Part model, mm, in its own coordinate system. A direction names the side the tool comes from. Coordinates: 2 decimals unless noted, no trailing zeros. Loops run counter-clockwise (first coordinate to the right, second up) from the corner with the lowest first, then second, coordinate; pieces in that order, holes last. Notation, with made-up numbers: M -39,-20 L -21,-20 A10 ccw -21,-12 Z; hole C -32,17.25 d8. An arc over 180 degrees is marked long. Answer as CSV lines item,"result". Start each with the question number.
from build123d import *

# Parameters (mm, degrees)
SKETCH061_W     = 19.99996
SKETCH061_H     = 48.49876
SKETCH061_R     = 1.7
PAD018_DEPTH    = 2.54
SKETCH038_W     = 20
SKETCH038_H     = 22.225
PAD004_DEPTH    = 1.5875
POCKET005_DEPTH = 12.7
POCKET006_DEPTH = 9.525
CHAMFER_SIZE    = 1.4986
SKETCH062_R     = 0.9
PAD019_DEPTH    = 2.975
CHAMFER002_SIZE = 1.016
CHAMFER005_SIZE = 1.58496


with BuildPart() as part:
    # Sketch061 → Pad018 (new body)
    with BuildSketch(Plane(origin=(0, 10, -45.999574), x_dir=(-1, 0, 0), z_dir=(0, 1, 0))):
        with Locations((0, 13.85062)):
            Rectangle(SKETCH061_W, SKETCH061_H)
        with Locations((-7.5, 5.00124)):
            Circle(SKETCH061_R, mode=Mode.SUBTRACT)
        with Locations((-7.5, -4.99876)):
            Circle(SKETCH061_R, mode=Mode.SUBTRACT)
        with Locations((7.5, -4.99876)):
            Circle(SKETCH061_R, mode=Mode.SUBTRACT)
        with Locations((7.5, 5.00124)):
            Circle(SKETCH061_R, mode=Mode.SUBTRACT)
    extrude(amount=PAD018_DEPTH)

    # Sketch038 (on Face10 of Pad018) → Pad004 (join)
    with BuildSketch(Plane(origin=(0, 12.54, -45.999574), x_dir=(-1, 0, 0), z_dir=(0, 1, 0))):
        with Locations((0, 26.9875)):
            Rectangle(SKETCH038_W, SKETCH038_H)
    extrude(amount=PAD004_DEPTH)

    # Sketch040 (on Face5 of Pad004) → Pocket005 (cut)
    with BuildSketch(Plane(origin=(0, 10, -7.899574), x_dir=(1, 0, 0), z_dir=(0, 0, 1))):
        Polygon((-2.184862, 4.1275), (0, 1.942638), (2.184862, 4.1275), align=None)
    extrude(amount=-POCKET005_DEPTH, mode=Mode.SUBTRACT)

    # Sketch037 (on Face18 of Pocket005) → Pocket006 (cut)
    with BuildSketch(Plane(origin=(0, 10, -20.599574), x_dir=(1, 0, 0), z_dir=(0, 0, 1))):
        with BuildLine():
            Line((-2.184862, 3.2225), (-2.184862, 4.1275))
            Line((-2.184862, 4.1275), (2.184862, 4.1275))
            Line((2.184862, 4.1275), (2.184862, 3.2225))
            ThreePointArc((-2.184862, 3.2225), (0, 1.037638), (2.184862, 3.2225))
        make_face()
    extrude(amount=-POCKET006_DEPTH, mode=Mode.SUBTRACT)

    # Chamfer
    chamfer_edges = [part.edges().sort_by_distance(p)[0] for p in [
        (0, 12.54, -30.124574),
    ]]
    chamfer(chamfer_edges, length=CHAMFER_SIZE)

    # Sketch062 (on Face6 of Chamfer) → Pad019 (join)
    with BuildSketch(Plane(origin=(0, 10, -56.398334), x_dir=(-1, 0, 0), z_dir=(0, 0, -1))):
        with BuildLine():
            Line((-3.175, 2.54), (-3.175, 0))
            Line((-3.175, 0), (3.175, 0))
            Line((3.175, 0), (3.175, 2.54))
            Line((3.175, 2.54), (1.90374, 6.488023))
            ThreePointArc((1.90374, 6.488023), (0, 7.87502), (-1.90374, 6.488023))
            Line((-1.90374, 6.488023), (-3.175, 2.54))
        make_face()
        with Locations((0, 5.87502)):
            Circle(SKETCH062_R, mode=Mode.SUBTRACT)
    extrude(amount=-PAD019_DEPTH)

    # Chamfer002
    chamfer002_edges = [part.edges().sort_by_distance(p)[0] for p in [
        (0, 12.54, -53.423334),
    ]]
    chamfer(chamfer002_edges, length=CHAMFER002_SIZE)

    # Chamfer005
    chamfer005_edges = [part.edges().sort_by_distance(p)[0] for p in [
        (6.092431, 14.1275, -30.124574),
        (-6.092431, 14.1275, -30.124574),
    ]]
    chamfer(chamfer005_edges, length=CHAMFER005_SIZE)


solid = part.part
Q1. Wall check: L1, parallel to Z at x = 7.5, y = 11.1; L2, parallel to Z at x = -6.75, y = 10.75; L3, parallel to Y at x = 2.5, z = -14.5. Give the ranges that are in metal, low to high.
Q2. Two-plate mould, pull along Z, no slides. Class faces 5 (the face through (0.1, 11.6, -7.9)), 6 (the face through (-0.5, 11.9, -20.6)), 7 (the face through (10, 11, -32)): +Z half, -Z half, draft (parallel to the pull), parting line (faces both ways), or undercut.
Q3. Tool access for faces 1 (the face through (-2.548, 14.486, -54.874)), 2 (the face through (2.53, 14.54, -54.87)), 3 (the face through (-1.11, 13.05, -14.16)), 4 (the face through (-2.185, 13.7, -25)): list every direction of +Z, -Z, +X, -X, +Y, -Y with a clear straight run to the whole face (end or side of a thin tool).
Q4. Slice it at A-A, the plane x = 7.5. State how many separate pieces and enclosed holes the cut face has, and give its area (3 significant figures).
Q5. Flat gauge pins, fed straight in: P1, Ø4, axis at x = 7.5, z = -51, coming from the +Y side; P2, Ø8, axis at x = 5.5, z = -26, coming from the +Y side; P3, Ø3, axis at x = -7.5, z = -51, coming from the +Y side; P4, Ø1, axis at x = 0.5, y = 13, coming from the +Z side. Where does each tip first touch, or does it go through?
Q6. Slice it at B-B, the plane z = -40.5. Write the cut outline in (x, y), and give its area (3 significant figures).
Solved:
1,L1,"z = -56.4 to -52.7, -49.3 to -42.7, -39.3 to -7.9"
1,L2,"z = -56.4 to -52.52, -49.47 to -42.52, -39.47 to -7.9"
1,L3,"y = 10 to 14.13"
2,face 5,"+Z half"
2,face 6,"undercut"
2,face 7,"draft"
3,face 1,"-Z, -X, +Y"
3,face 2,"-Z, +X, +Y"
3,face 3,"+Z, +Y"
3,face 4,"+Y"
4,separate pieces,"3"
4,enclosed holes,"0"
4,area,"140 mm2"
5,P1,"stops at y = 12.54"
5,P2,"stops at y = 14.13"
5,P3,"passes through"
5,P4,"stops at z = -7.9"
6,outline,"M -10,10 L -9.13,10 L -9.13,12.54 L -10,12.54 Z; M -5.87,10 L 5.87,10 L 5.87,12.54 L -5.87,12.54 Z; M 9.13,10 L 10,10 L 10,12.54 L 9.13,12.54 Z"
6,area,"34.3 mm2"
